Design review of the part built by this model. Coordinates are the model's own, in mm. Round coordinates to 2 decimals unless told otherwise and drop trailing zeros. Loops run counter-clockwise (first coordinate to the right, second up) from the corner with the lowest first, then second, coordinate; pieces in that order, holes last. Notation, with made-up numbers: (-39.5, -39.75) - (-9.5, -39.75) arc R16 ccw to (-9.5, -17.75) - close; hole circle Ø1 at (4.25, -20.5). An arc over 180 degrees is marked (long way). Answer as CSV lines item,"result". Start each with the question number.
(1) Mouldability with a two-part tool opening along Y and no side actions: class faces 1 (the flat face through (-3, 0, -153)), 2 (the cylindrical face through (-19.527, -29.58, 148.724)), 3 (the cylindrical face through (225.49, -15.19, -50.07)) as released by +Y, released by -Y, zero draft, split by the parting line, or undercut.
(2) For P1, Ø3, axis at x = -80, z = 145, coming from the +Y side; P2, Ø10, axis at y = -36, z = 166.5, coming from the -X side; P3, Ø4, axis at y = -23.5, z = -127.5, coming from the -X side; P4, Ø4, axis at y = -36, z = 156.5, coming from the +X side, all flat-tipped, find the tip position at first contact; note any pin that passes through.
(3) Consider section C-C (y = -35). Give the boundary of the cut face in (x, z).
(4) Wall thickness on L1, parallel to Z at x = 0, y = -22; L2, parallel to Z at x = 0, y = -14; L3, parallel to X at y = -38.5, z = -29: over which ranges is each line inside the solid? List them lowest first.
from build123d import *

# Parameters (mm, degrees)
F0_R     = 235
F0_R_2   = 150
F1_DEPTH = 60


with BuildPart() as f1:
    # F0 (on Front) → F1 (new body)
    with BuildSketch(Plane.XZ):
        Circle(F0_R)
        Circle(F0_R_2, mode=Mode.SUBTRACT)
    extrude(amount=F1_DEPTH)

    # F2 (on Right) → F3 (revolve, cut)
    with BuildSketch(Plane.YZ):
        with BuildLine():
            Line((-17.486282, 236.367822), (-17.452006, 234.98348))
            Line((-17.452006, 234.98348), (-18.446662, 233.260686))
            ThreePointArc((-18.446662, 233.260686), (-18.446662, 231.740686), (-17.130303, 230.980686))
            Line((-17.130303, 230.980686), (-15.217006, 230.980686))
            Line((-15.217006, 230.980686), (-13.303709, 230.980686))
            ThreePointArc((-13.303709, 230.980686), (-11.98735, 231.740686), (-11.98735, 233.260686))
            Line((-11.98735, 233.260686), (-12.982006, 234.98348))
            Line((-12.982006, 234.98348), (-12.982006, 236.367822))
            Line((-12.982006, 236.367822), (-17.486282, 236.367822))
        make_face()
    revolve(axis=Axis((0, -68.413801, 0), (0, -1, 0)), mode=Mode.SUBTRACT)


solid = f1.part
Determined:
1,face 1,"released by +Y"
1,face 2,"zero draft"
1,face 3,"undercut"
2,P1,"stops at y = 0"
2,P2,"stops at x = -170.71"
2,P3,"stops at x = -198.68"
2,P4,"stops at x = 177.07"
3,outline,"circle Ø470 at (0, 0); hole circle Ø300 at (0, 0)"
4,L1,"z = -235 to -150, 150 to 235"
4,L2,"z = -230.98 to -150, 150 to 230.98"
4,L3,"x = -233.2 to -147.17, 147.17 to 233.2"
